```python
from build123d import *

# Parameters (mm, degrees)
F0_W     = 203.2
F0_H     = 203.2
F1_DEPTH = 177.8
F3_DEPTH = 177.8
F4_W     = 203.2
F4_H     = 152.4
F5_DEPTH = 127
F6_DEPTH = 127


with BuildPart() as f1:
    # F0 (on Front) → F1 (new body)
    with BuildSketch(Plane.XZ):
        Rectangle(F0_W, F0_H)
    extrude(amount=F1_DEPTH)

    # F2 (on face) → F3 (join)
    with BuildSketch(Plane(origin=(0, 0, 0), x_dir=(-1, 0, 0), z_dir=(0, 1, 0))):
        Polygon((0, 203.2), (-101.6, 101.6), (101.6, 101.6), align=None)
    extrude(amount=-F3_DEPTH)

    # F4 (on face) → F5 (join)
    with BuildSketch(Plane.XZ.offset(177.8)):
        with Locations((0, -25.4)):
            Rectangle(F4_W, F4_H)
    extrude(amount=F5_DEPTH)

    # F4 (on face) → F6 (join)
    with BuildSketch(Plane.XZ.offset(177.8)):
        Polygon((-101.6, 101.6), (-101.6, 50.8), (101.6, 50.8), (101.6, 101.6), (0, 203.2), align=None)
        Polygon((0, 203.2), (101.6, 101.6), (101.6, 152.4), align=None)
    extrude(amount=F6_DEPTH)


solid = f1.part
```
Input: part model. Units: mm. Frame: model coordinates. A direction names the side the tool comes from. Coordinates: 2 decimals unless noted, no trailing zeros. Loops run counter-clockwise (first coordinate to the right, second up) from the corner with the lowest first, then second, coordinate; pieces in that order, holes last. Notation, with made-up numbers: (-23.5, -10.75) -> (25.5, -10.75) arc R29 cw to (25.5, 14.25) -> close; hole circle Ø2 at (61, 9.5). An arc over 180 degrees is marked (long way). Use a Markdown table: item, result.
1) Cut plane D-D (y = -193.5). Return the cut outline in (x, z), then the cut area to 3 significant figures.
Results found:
| item | result |
|---|---|
| outline | (-101.6, -101.6) -> (101.6, -101.6) -> (101.6, 152.4) -> (0, 203.2) -> (-101.6, 101.6) -> close |
| area | 54,200 mm2 |
2) Material intervals for line 1 along Y through (x, z) = (66.5, 152); line 2 along Z through (x, y) = (75, -70); line 3 along Z through (x, y) = (70, -199.5), sorted ascending. Write a range as from..to.
Results found:
| item | result |
|---|---|
| line 1 | y = -304.8..-177.8 |
| line 2 | z = -101.6..128.2 |
| line 3 | z = -101.6..168.2 |
3) Cut plane A-A (x = 33). Return the cut outline in (y, z), then the cut area to 3 significant figures.
Results found:
| item | result |
|---|---|
| outline | (-304.8, -101.6) -> (0, -101.6) -> (0, 170.2) -> (-177.8, 170.2) -> (-177.8, 186.7) -> (-304.8, 186.7) -> close |
| area | 84,900 mm2 |
4) Access query for faces 1 (the flat face through (-50.1, -150.3, 153.1)), 2 (the flat face through (50.1, -87.7, 153.1)). Directions: +Z, -Z, +X, -X, +Y, -Y. A direction counts if a zero-diameter tool reaches every point of the face in a straight line with its end or side. Return the directions, or none.
Results found:
| item | result |
|---|---|
| face 1 | +Z, -X, +Y, -Y |
| face 2 | +Z, +X, +Y |
5) Cut plane B-B (z = 157). Return the cut outline in (x, y).
Results found:
| item | result |
|---|---|
| outline | (-46.2, -304.8) -> (92.4, -304.8) -> (92.4, -177.8) -> (46.2, -177.8) -> (46.2, 0) -> (-46.2, 0) -> close |
6) Cut plane C-C (y = -141.5). Return the cut outline in (x, z).
Results found:
| item | result |
|---|---|
| outline | (-101.6, -101.6) -> (101.6, -101.6) -> (101.6, 101.6) -> (0, 203.2) -> (-101.6, 101.6) -> close |
